from build123d import *

# Parameters (mm, degrees)
SKETCH_1_R          = 3.5
EXTRUDE_1_DEPTH     = 2
SKETCH_2_W          = 0.799406376
SKETCH_2_H          = 7.454929226
CUT_EXTRUDE_1_DEPTH = 1
SKETCH_3_R          = 1.5
EXTRUDE_2_DEPTH     = 5
CHAMFER_1_SIZE      = 1


with BuildPart() as part:
    # Эскиз1 → Бобышка-Вытянуть1 (new body)
    with BuildSketch(Plane.XY):
        Circle(SKETCH_1_R)
    extrude(amount=EXTRUDE_1_DEPTH)

    # Эскиз2 → Вырез-Вытянуть1 (cut)
    with BuildSketch(Plane.XY.offset(2)):
        Rectangle(SKETCH_2_W, SKETCH_2_H)
    extrude(amount=-CUT_EXTRUDE_1_DEPTH, mode=Mode.SUBTRACT)

    # Эскиз3 → Бобышка-Вытянуть2 (add)
    with BuildSketch(Plane(origin=(0, 0, 0), x_dir=(-1, 0, 0), z_dir=(0, 0, -1))):
        Circle(SKETCH_3_R)
    extrude(amount=EXTRUDE_2_DEPTH)

    # Фаска1
    chamfer_1_edges = [part.edges().sort_by_distance(p)[0] for p in [
        (1.5, 0, -5),
    ]]
    chamfer(chamfer_1_edges, length=CHAMFER_1_SIZE)

    # Эскиз6 → Вырез-Повернуть3 (revolve, cut)
    with BuildSketch(Plane(origin=(0, 0, 0), x_dir=(1, 0, 0), z_dir=(0, 1, 0))):
        with BuildLine():
            Line((0.1, -2), (3.503572085, -2))
            Line((3.503572085, -2), (3.503572085, -1.195824387))
            ThreePointArc((3.503572085, -1.195824387), (1.848642427, -1.796225946), (0.1, -2))
        make_face()
    revolve(axis=Axis((0, 0, 4.44135275), (0, 0, -1)), mode=Mode.SUBTRACT)


solid = part.part
Work out the finished part from the listing and answer in its coordinate system (mm). Give positions to 0.01 mm unless a question says otherwise; leave off trailing zeros. Write each loop counter-clockwise with the first axis right and the second up, starting at its lowest first coordinate (ties: lowest second). Pieces come first, ordered by that corner, then holes.
Q1. The part is cut by section B-B on z = 0.5. Give the vertices of the cut face in (x, y), and give its area (3 significant figures).
Answer:
outline: circle Ø7 at (0, 0)
area: 38.5 mm2
Q2. The part is cut by section A-A on x = 0. Give the vertices of the cut face in (y, z).
Answer:
outline: (-3.5, 0) - (-1.5, 0) - (-1.5, -4) - (-0.5, -5) - (0.5, -5) - (1.5, -4) - (1.5, 0) - (3.5, 0) - (3.5, 1) - (-3.5, 1) - close
Q3. Straight lines are drawn through the part: L1, parallel to Y at x = 0, z = -3; L2, parallel to Y at x = 0.75, z = 0.75; L3, parallel to Z at x = 2.25, y = 1.5. For each, find the intervals that lie inside material, in ascending order.
Answer:
L1: y = -1.5 to 1.5
L2: y = -3.42 to 3.42
L3: z = 0 to 1.54
Q4. Given pin 1 (3 mm diameter, centred on x = 2, z = -4, fed in from -Y); pin 2 (4 mm diameter, centred on x = 0, y = -2.5, fed in from +Z); pin 3 (3 mm diameter, centred on y = 1, z = -3.5, fed in from +X), each flat-ended and moving along its own axis, determine where each tip first touches the part or whether it passes through.
Answer:
pin 1: stops at y = -1.41
pin 2: stops at z = 1.98
pin 3: stops at x = 1.5
Q5. For a pull along X with two mould halves and no side action, classify faces 1 (the face through (0.4, 0, 1.4)), 2 (the face through (-0.4, 0, 1.4)), 3 (the face through (3.233, -1.341, 0.59)), 4 (the face through (0, 0, -5)) as released by +X, released by -X, zero draft, split by the parting line, or undercut.
Answer:
face 1: undercut
face 2: undercut
face 3: split by the parting line
face 4: zero draft
Q6. The part is cut by section C-C on z = -2.25. Give the vertices of the cut face in (x, y), and give its area (3 significant figures).
Answer:
outline: circle Ø3 at (0, 0)
area: 7.07 mm2
